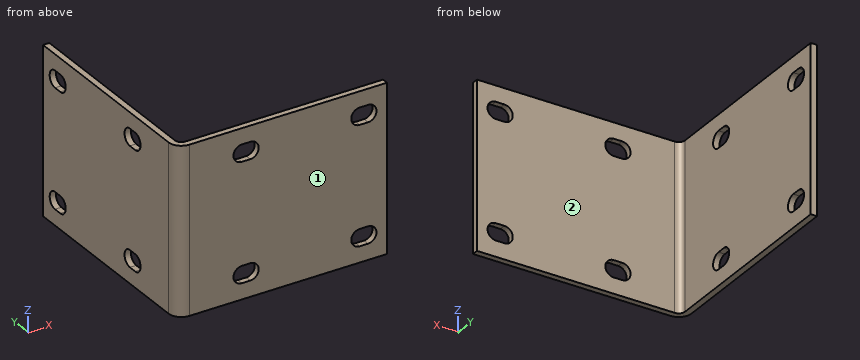
from build123d import *

# Parameters (mm, degrees)
BOSS_EXTRUDE1_DEPTH = 62.70625
CUT_EXTRUDE1_DEPTH  = 224.410663511


with BuildPart() as part:
    # Sketch1 → Boss-Extrude1 (new, symmetric)
    with BuildSketch(Plane.XY):
        with BuildLine():
            Line((-9.525, 149.225), (-4.7625, 149.225))
            Line((-4.7625, 149.225), (-4.7625, 0))
            ThreePointArc((-4.7625, 0), (-3.367596045, -3.367596045), (0, -4.7625))
            Line((0, -4.7625), (149.225, -4.7625))
            Line((149.225, -4.7625), (149.225, -9.525))
            Line((149.225, -9.525), (0, -9.525))
            ThreePointArc((0, -9.525), (-6.735192091, -6.735192091), (-9.525, 0))
            Line((-9.525, 0), (-9.525, 149.225))
        make_face()
    extrude(amount=BOSS_EXTRUDE1_DEPTH, both=True)

    # Sketch2 → Cut-Extrude1 (cut, through all)
    with BuildSketch(Plane(origin=(-4.7625, 0, 0), x_dir=(0, 0, -1), z_dir=(1, 0, 0))):
        with BuildLine():
            Line((-50.8, 134.9375), (-50.8, 128.5875))
            ThreePointArc((-50.8, 128.5875), (-44.45, 122.2375), (-38.1, 128.5875))
            Line((-38.1, 128.5875), (-38.1, 134.9375))
            ThreePointArc((-38.1, 134.9375), (-44.45, 141.2875), (-50.8, 134.9375))
        make_face()
        with BuildLine():
            Line((-50.8, 46.0375), (-50.8, 39.6875))
            ThreePointArc((-50.8, 39.6875), (-44.45, 33.3375), (-38.1, 39.6875))
            Line((-38.1, 39.6875), (-38.1, 46.0375))
            ThreePointArc((-38.1, 46.0375), (-44.45, 52.3875), (-50.8, 46.0375))
        make_face()
        with BuildLine():
            Line((38.1, 39.6875), (38.1, 46.0375))
            ThreePointArc((38.1, 46.0375), (44.45, 52.3875), (50.8, 46.0375))
            Line((50.8, 46.0375), (50.8, 39.6875))
            ThreePointArc((50.8, 39.6875), (44.45, 33.3375), (38.1, 39.6875))
        make_face()
        with BuildLine():
            Line((38.1, 134.9375), (38.1, 128.5875))
            ThreePointArc((38.1, 128.5875), (44.45, 122.2375), (50.8, 128.5875))
            Line((50.8, 128.5875), (50.8, 134.9375))
            ThreePointArc((50.8, 134.9375), (44.45, 141.2875), (38.1, 134.9375))
        make_face()
    cut_extrude1 = extrude(amount=-CUT_EXTRUDE1_DEPTH, mode=Mode.SUBTRACT)

    # Mirror1: Cut-Extrude1 across plane
    add(cut_extrude1.mirror(Plane(origin=(0, 0, 0), x_dir=(0, 0, 1), z_dir=(0.7071067811865475, -0.7071067811865476, 0))), mode=Mode.SUBTRACT)


solid = part.part
Verification items for the finished model (mm, model axes). Face numbers are marked on the shaded views. A direction names the side the tool comes from. Coordinates: 2 decimals unless noted, no trailing zeros. Write each loop counter-clockwise with the first axis right and the second up, starting at its lowest first coordinate (ties: lowest second). Pieces come first, ordered by that corner, then holes. Notation, with made-up numbers: (16, -38.5) -> (26, -38.5) arc R17 cw to (26, -19.5) -> close; hole circle Ø10 at (-12, -15). An arc over 180 degrees is marked (long way). One line per item, written item: value. Start each with the question number.
Q1. Cross-section at B-B on x = 132. Enter the section's corners in (y, z) (1 decimal), and give its area (3 significant figures).
Q2. Go/stop test with a flat-tipped pin: P1, Ø1, axis at y = 88, z = 16.5, coming from the +X side. Record where the tip stops, or that it passes through.
Q3. Access from +Z, -Z, +X, -X, +Y, -Y to the whole of each face (thin tool, end or side, straight path). Record for the marked faces 1 and 2.
Q4. Cross-section at D-D on y = 94. Enter the section's corners in (x, z) (1 decimal).
Q5. Thickness scan on L1, parallel to X at y = 29, z = -37 (1 decimal); L2, parallel to X at y = -2.5, z = -1.5. Record the ranges inside material, lowest first. Write a range as from..to.
Q6. Cross-section at A-A on z = -44.45. State how many separate pieces and enclosed holes the cut face has, and give its area (3 significant figures).
Checked values:
1. outline: (-9.5, -62.7) -> (-4.8, -62.7) -> (-4.8, -50.8) -> (-9.5, -50.8) -> close; (-9.5, -38.1) -> (-4.8, -38.1) -> (-4.8, 38.1) -> (-9.5, 38.1) -> close; (-9.5, 50.8) -> (-4.8, 50.8) -> (-4.8, 62.7) -> (-9.5, 62.7) -> close
1. area: 476 mm²
2. P1: stops at x = -4.76
3. face 1: +Z, -Z, +X, -X, -Y
3. face 2: +Z, -Z, +X, +Y
4. outline: (-9.5, -62.7) -> (-4.8, -62.7) -> (-4.8, 62.7) -> (-9.5, 62.7) -> close
5. L1: x = -9.5..-4.8
5. L2: x = -9.19..-4.05
6. separate pieces: 5
6. enclosed holes: 0
6. area: 1,110 mm²
